```python
from build123d import *

# Parameters (mm, degrees)
SKETCH_1_W          = 970
SKETCH_1_H          = 200
SKETCH_1_W_2        = 940
SKETCH_1_H_2        = 170
EXTRUDE_1_DEPTH     = 200
SKETCH_2_W          = 970
SKETCH_2_H          = 200
EXTRUDE_2_DEPTH     = 10
SKETCH_3_W          = 250
SKETCH_3_H          = 30
EXTRUDE_3_DEPTH     = 120
SKETCH_4_W          = 200
SKETCH_4_H          = 95
CUT_EXTRUDE_1_DEPTH = 120
CHAMFER_1_SIZE      = 10
CHAMFER_2_SIZE      = 50


with BuildPart() as part:
    # 草图1 → 凸台-拉伸1 (new body)
    with BuildSketch(Plane(origin=(0, 0, 0), x_dir=(1, 0, 0), z_dir=(0, 1, 0))):
        Rectangle(SKETCH_1_W, SKETCH_1_H)
        Rectangle(SKETCH_1_W_2, SKETCH_1_H_2, mode=Mode.SUBTRACT)
    extrude(amount=EXTRUDE_1_DEPTH)

    # 草图2 → 凸台-拉伸2 (add)
    with BuildSketch(Plane.XZ):
        Rectangle(SKETCH_2_W, SKETCH_2_H)
    extrude(amount=EXTRUDE_2_DEPTH)

    # 草图3 → 凸台-拉伸3 (add)
    with BuildSketch(Plane(origin=(0, 0, -100), x_dir=(-1, 0, 0), z_dir=(0, 0, -1))):
        with Locations((0, 95)):
            Rectangle(SKETCH_3_W, SKETCH_3_H)
    extrude(amount=EXTRUDE_3_DEPTH)

    # 草图4 → 切除-拉伸1 (cut)
    with BuildSketch(Plane(origin=(0, 110, 0), x_dir=(1, 0, 0), z_dir=(0, 1, 0))):
        with Locations((0, 147.5)):
            Rectangle(SKETCH_4_W, SKETCH_4_H)
    extrude(amount=-CUT_EXTRUDE_1_DEPTH, mode=Mode.SUBTRACT)

    # 倒角1
    chamfer_1_edges = [part.edges().sort_by_distance(p)[0] for p in [
        (-125, 95, -100),
        (-112.5, 110, -100),
        (125, 95, -100),
        (112.5, 80, -100),
        (-112.5, 80, -100),
        (112.5, 110, -100),
        (-100, 95, -100),
        (100, 95, -100),
    ]]
    chamfer(chamfer_1_edges, length=CHAMFER_1_SIZE)

    # 倒角2
    chamfer_2_edges = [part.edges().sort_by_distance(p)[0] for p in [
        (-125, 95, -220),
        (125, 95, -220),
        (-100, 95, -195),
        (100, 95, -195),
    ]]
    chamfer(chamfer_2_edges, length=CHAMFER_2_SIZE)


solid = part.part
```
Geometry check sheet. Reference: the model listing, model coordinates, mm. A direction names the side the tool comes from. Give positions to 0.01 mm unless a question says otherwise; leave off trailing zeros. Write each loop counter-clockwise with the first axis right and the second up, starting at its lowest first coordinate (ties: lowest second). Pieces come first, ordered by that corner, then holes.
1) Section check A-A, the plane x = 15. Record the boundary of the cut face in (y, z).
2) Material ranges on L1, parallel to Z at x = -294, y = 72; L2, parallel to X at y = 22.5, z = 25; L3, parallel to X at y = 85, z = -127.5, recorded low to high.
3) Section check D-D, the plane x = 115. Record the boundary of the cut face in (y, z), and give its area (3 significant figures).
4) Release check for a two-part mould opening along X. For faces 1 (the flat face through (-7, 96, 100)), 2 (the flat face through (-470, 99, 1)), 3 (the flat face through (100, 95, -195)) record: pulls with the +X half, pulls with the -X half, needs draft (parallel to the pull), parting line crosses it, or undercut.
5) Section check B-B, the plane z = -130.5. Record the boundary of the cut face in (x, y).
6) Section check C-C, the plane y = 151. Record the boundary of the cut face in (x, z), and give its area (3 significant figures).
7) Access from +Z, -Z, +X, -X, +Y, -Y to the whole of each face (thin tool, end or side, straight path). Record for faces 4 (the flat face through (-125, 95, -140)), 5 (the flat face through (-75, 95, -170)), 6 (the flat face through (2, 80, -201)), 7 (the flat face through (2, 110, -201)), 8 (the flat face through (-7, 99, -85)).
8) Gauge pin test, flat ends, axial feed: pin 1 (9 mm diameter, centred on y = 93.5, z = -136, fed in from -X); pin 2 (8 mm diameter, centred on x = 50, z = 50.5, fed in from +Y); pin 3 (5 mm diameter, centred on x = -123.5, y = 32, fed in from -Z). Record the tip position at first contact, or that the pin passes through.
Computed:
1. outline: (-10, -100) - (200, -100) - (200, -85) - (0, -85) - (0, 85) - (200, 85) - (200, 100) - (-10, 100) - close; (80, -220) - (110, -220) - (110, -195) - (80, -195) - close
2. L1: z = -100 to -85, 85 to 100
2. L2: x = -485 to -470, 470 to 485
2. L3: x = -125 to -100, 100 to 125
3. outline: (-10, -100) - (70, -100) - (80, -110) - (80, -180) - (110, -180) - (110, -110) - (120, -100) - (200, -100) - (200, -85) - (0, -85) - (0, 85) - (200, 85) - (200, 100) - (-10, 100) - close
3. area: 10,500 mm2
4. face 1: needs draft
4. face 2: undercut
4. face 3: pulls with the +X half
5. outline: (-125, 80) - (-100, 80) - (-100, 110) - (-125, 110) - close; (100, 80) - (125, 80) - (125, 110) - (100, 110) - close
6. outline: (-485, -100) - (485, -100) - (485, 100) - (-485, 100) - close; hole (-470, -85) - (470, -85) - (470, 85) - (-470, 85) - close
6. area: 34,200 mm2
7. face 4: -Z, -X, +Y, -Y
7. face 5: +Y, -Y
7. face 6: -Z, +X, -X, -Y
7. face 7: -Z, +X, -X, +Y
7. face 8: +Y
8. pin 1: stops at x = -125
8. pin 2: stops at y = 0
8. pin 3: stops at z = -100
